Geometry: final body of the model. Coordinates: model frame, mm. Face numbers are marked on the shaded views. A direction names the side the tool comes from. Round coordinates to 2 decimals unless told otherwise and drop trailing zeros. Write each loop counter-clockwise with the first axis right and the second up, starting at its lowest first coordinate (ties: lowest second). Pieces come first, ordered by that corner, then holes. Notation, with made-up numbers: M -28,-28.5 L 27,-28.5 A21 cw 27,-15.5 Z; hole C 47,84 d3. An arc over 180 degrees is marked long. Use one line per item in the form item = value. Start each with the question number.
Item 1: Pin query (flat end, axial travel): pin 1 Ø19 at (x, z) = (17.5, 32) entering from -Y; pin 2 Ø12 at (x, z) = (2.5, 23.5) entering from -Y; pin 3 Ø6 at (y, z) = (12.8, 34) entering from -X; pin 4 Ø4 at (x, z) = (3, 16) entering from -Y. Return the tip coordinate at first contact, or that it passes through.
Item 2: Section query C-C (y = 33.5). Return loops of the section in (x, z).
Item 3: Pull-direction query (X, two-part tool) for the marked faces 3, 4 and 5; classes: pulls with the +X half, pulls with the -X half, needs draft (parallel to the pull), parting line crosses it, or undercut.
Item 4: Section query D-D (z = 33). Return loops of the section in (x, y), and give its area (3 significant figures).
Item 5: Section query A-A (x = 16.61). Return loops of the section in (y, z), and give its area (3 significant figures).
Item 6: Section query B-B (z = 21). Return loops of the section in (x, y), and give its area (3 significant figures).
Item 7: Ray query, probe 1 along X at (y, z) = (44.5, 33); probe 2 along Y at (x, z) = (20, 39.5); probe 3 along X at (y, z) = (69, 39). Return the intervals inside material, ascending.
Item 8: Reachability of the marked faces 1 and 2 from +Z, -Z, +X, -X, +Y, -Y: full face, straight path, thin tool, end or side. Return the list, or none.
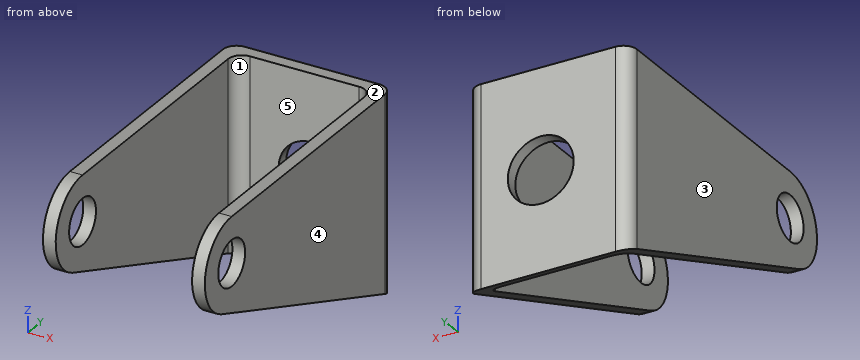
from build123d import *

# Parameters (mm, degrees)
EXTRUDE_THIN1_DEPTH = 44
SKETCH3_OUTSIDE_W   = 64.442
SKETCH3_OUTSIDE_H   = 93.242
CUT_EXTRUDE1_DEPTH  = 93.212797377
SKETCH4_R           = 5
CUT_EXTRUDE2_DEPTH  = 93.212797377
SKETCH5_R           = 7.25
CUT_EXTRUDE3_DEPTH  = 10
FILLET3_R           = 3


with BuildPart() as part:
    # Sketch1 → Extrude-Thin1 (new body)
    with BuildSketch(Plane.XY):
        Polygon((0, 0), (0, 70), (30, 70), (30, 0), (32.8, 0), (32.8, 72.8), (-2.8, 72.8), (-2.8, 0), align=None)
    extrude(amount=EXTRUDE_THIN1_DEPTH)

    # Sketch3 outside → Cut-Extrude1 (cut, through all)
    with BuildSketch(Plane(origin=(32.8, 0, 0), x_dir=(0, 0, -1), z_dir=(1, 0, 0))):
        with Locations((-22, 36.4)):
            Rectangle(SKETCH3_OUTSIDE_W, SKETCH3_OUTSIDE_H)
        with BuildLine():
            Line((-44, 12.8), (-44, 72.8))
            Line((-44, 72.8), (0, 72.8))
            Line((0, 72.8), (-24.676843343, 9.183544561))
            ThreePointArc((-24.676843343, 9.183544561), (-35.839624069, 2.9706672), (-44, 12.8))
        make_face(mode=Mode.SUBTRACT)
    extrude(amount=-CUT_EXTRUDE1_DEPTH, mode=Mode.SUBTRACT)

    # Sketch4 → Cut-Extrude2 (cut, through all)
    with BuildSketch(Plane.ZY.offset(2.8)):
        with Locations((34, 12.8)):
            Circle(SKETCH4_R)
    extrude(amount=-CUT_EXTRUDE2_DEPTH, mode=Mode.SUBTRACT)

    # Sketch5 → Cut-Extrude3 (cut)
    with BuildSketch(Plane(origin=(0, 72.8, 0), x_dir=(1, 0, 0), z_dir=(0, 1, 0))):
        with Locations(Location((16.61, -22, 0), (0, 0, 270))):
            Circle(SKETCH5_R)
    extrude(amount=-CUT_EXTRUDE3_DEPTH, mode=Mode.SUBTRACT)

    # Fillet3
    fillet3_edges = [part.edges().sort_by_distance(p)[0] for p in [
        (30, 70, 22.543060446),
        (0, 70, 22.543060446),
        (-2.8, 72.8, 22),
        (32.8, 72.8, 22),
    ]]
    fillet(fillet3_edges, radius=FILLET3_R)


solid = part.part
Working result:
q1.pin_1 = 70
q1.pin_2 = 4.17
q1.pin_3 = through
q1.pin_4 = 69.24
q2.outline = M -2.8,15.24 L 0,15.24 L 0,44 L -2.8,44 Z; M 30,15.24 L 32.8,15.24 L 32.8,44 L 30,44 Z
q3.face_3 = pulls with the -X half
q3.face_4 = pulls with the +X half
q3.face_5 = undercut
q4.outline = M -2.8,2.85 L 0,2.85 L 0,7.9 L -2.8,7.9 Z; M -2.8,17.7 L 0,17.7 L 0,67 A3 cw 3,70 L 27,70 A3 cw 30,67 L 30,17.7 L 32.8,17.7 L 32.8,69.8 A3 ccw 29.8,72.8 L 0.2,72.8 A3 ccw -2.8,69.8 Z; M 30,2.85 L 32.8,2.85 L 32.8,7.9 L 30,7.9 Z
q4.area = 421 mm²
q5.outline = M 70,1.09 L 72.8,0 L 72.8,14.75 L 70,14.75 Z; M 70,29.25 L 72.8,29.25 L 72.8,44 L 70,44 Z
q5.area = 81.1 mm²
q6.outline = M -2.8,18.66 L 0,18.66 L 0,67 A3 cw 3,70 L 9.43,70 L 9.43,72.8 L 0.2,72.8 A3 ccw -2.8,69.8 Z; M 23.79,70 L 27,70 A3 cw 30,67 L 30,18.66 L 32.8,18.66 L 32.8,69.8 A3 ccw 29.8,72.8 L 23.79,72.8 Z
q6.area = 347 mm²
q7.probe_1 = -2.8 to 0, 30 to 32.8
q7.probe_2 = 70 to 72.8
q7.probe_3 = -2.8 to 0.76, 29.24 to 32.8
q8.face_1 = +Z, -Z, -Y
q8.face_2 = +Z, +X, -X, +Y, -Y
